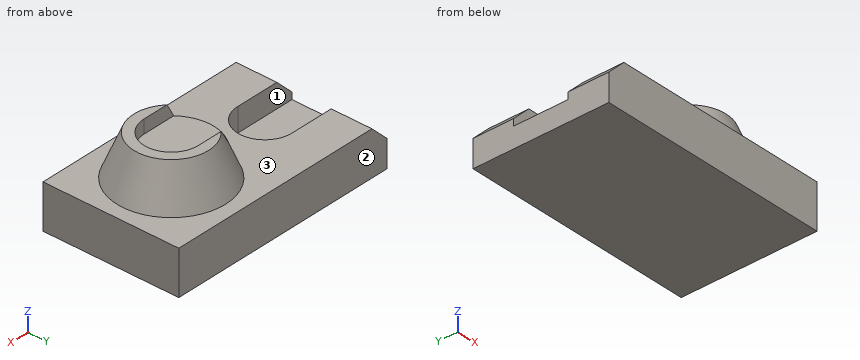
```python
from build123d import *

# Parameters (mm, degrees)
F0_W     = 109.5375
F0_H     = 63.5
F1_DEPTH = 20.6502
F5_DEPTH = 6.35
F7_DEPTH = 11.1252
F8_SIZE  = 7.9375


with BuildPart() as f1:
    # F0 (on Top) → F1 (new body)
    with BuildSketch(Plane.XY):
        with Locations((-23.01875, 0)):
            Rectangle(F0_W, F0_H)
    extrude(amount=F1_DEPTH)

    # F2 (on Right) → F3 (revolve)
    with BuildSketch(Plane.YZ):
        Polygon((0, 20.6502), (25.4, 20.6502), (17.4625, 39.7002), (0, 39.7002), align=None)
    revolve(axis=Axis((0, 0, 30.1752), (0, 0, -1)))

    # F4 (on face) → F5 (cut)
    with BuildSketch(Plane.XY.offset(39.7002)):
        with BuildLine():
            Line((-30.736892, -12.7), (-11.985362, -12.7))
            ThreePointArc((-11.985362, -12.7), (-17.4625, 0), (-11.985362, 12.7))
            Line((-11.985362, 12.7), (-30.736892, 12.7))
            Line((-30.736892, 12.7), (-30.736892, -12.7))
        make_face()
        with BuildLine():
            Line((-11.985362, -12.7), (0, -12.7))
            ThreePointArc((0, -12.7), (12.7, 0), (0, 12.7))
            Line((0, 12.7), (-11.985362, 12.7))
            ThreePointArc((-11.985362, 12.7), (-17.4625, 0), (-11.985362, -12.7))
        make_face()
    extrude(amount=-F5_DEPTH, mode=Mode.SUBTRACT)

    # F6 (on face) → F7 (cut)
    with BuildSketch(Plane.XY.offset(20.6502)):
        with BuildLine():
            Line((-77.7875, -12.697648), (-49.456894, -12.697648))
            ThreePointArc((-49.456894, -12.697648), (-36.512501, -0.004972), (-49.446951, 12.697836))
            Line((-49.446951, 12.697836), (-77.7875, 12.697836))
            Line((-77.7875, 12.697836), (-77.7875, -12.697648))
        make_face()
    extrude(amount=-F7_DEPTH, mode=Mode.SUBTRACT)

    # F8
    f8_edges = [f1.edges().sort_by_distance(p)[0] for p in [
        (-77.7875, -22.223824, 20.6502),
        (-77.7875, 22.223918, 20.6502),
    ]]
    chamfer(f8_edges, length=F8_SIZE)


solid = f1.part
```
Could you check a few things on this model? Use its own coordinates, in mm. Face numbers are marked on the shaded views. A direction names the side the tool comes from. Give positions to 0.01 mm unless a question says otherwise; leave off trailing zeros. Order: outer loops, then holes, each group sorted by start corner. A loop starts at its lowest first (then second) coordinate and runs counter-clockwise, first axis right, second up.
Q1. Suppose I cut it at B-B, the plane z = 15. Write out the boundary of the cut face in (x, y).
Q2. If I drill on line 1 along Y through (x, z) = (-72.5, 13); line 2 along Z through (x, y) = (-28, 25); line 3 along Z through (x, y) = (9, -2), over which ranges is the centre line in solid material (lowest first)?
Q3. Suppose I cut it at D-D, the plane z = 30. Write out the boundary of the cut face in (x, y), and give its area (3 significant figures).
Q4. I'm going to push flat-ended pins straight in: P1, Ø5, axis at x = -7.5, z = 38, coming from the -Y side; P2, Ø7.5, axis at x = -10, y = 0, coming from the +Z side; P3, Ø5, axis at x = 16.5, z = 29, coming from the +Y side. Where does each tip first touch, or does it pass through?
Q5. Suppose I cut it at C-C, the plane x = -44. Write out the boundary of the cut face in (y, z) (3 decimals), and give its area (3 significant figures).
Q6. For the marked faces 1, 2 and 3, which set-ups out of +Z, -Z, +X, -X, +Y, -Y let a thin tool reach every point of the face, with its end or its side?
Solution:
1. outline: (-75.5, -31.75) - (31.75, -31.75) - (31.75, 31.75) - (-75.5, 31.75) - (-75.5, 12.7) - (-49.45, 12.7) arc R12.7 cw (long way) to (-49.46, -12.7) - (-75.5, -12.7) - close
2. line 1: y = -31.75 to -12.7, 12.7 to 31.75
2. line 2: z = 0 to 20.65
2. line 3: z = 0 to 33.35
3. outline: circle Ø43.01 at (0, 0)
3. area: 1,450 mm2
4. P1: stops at y = -18.03
4. P2: stops at z = 33.35
4. P3: stops at y = 17.27
5. outline: (-31.75, 0) - (31.75, 0) - (31.75, 20.65) - (11.581, 20.65) - (11.581, 9.525) - (-11.581, 9.525) - (-11.581, 20.65) - (-31.75, 20.65) - close
5. area: 1,050 mm2
6. face 1: +Z, -X
6. face 2: +Z, -Z, +X, -X, +Y
6. face 3: +Z
